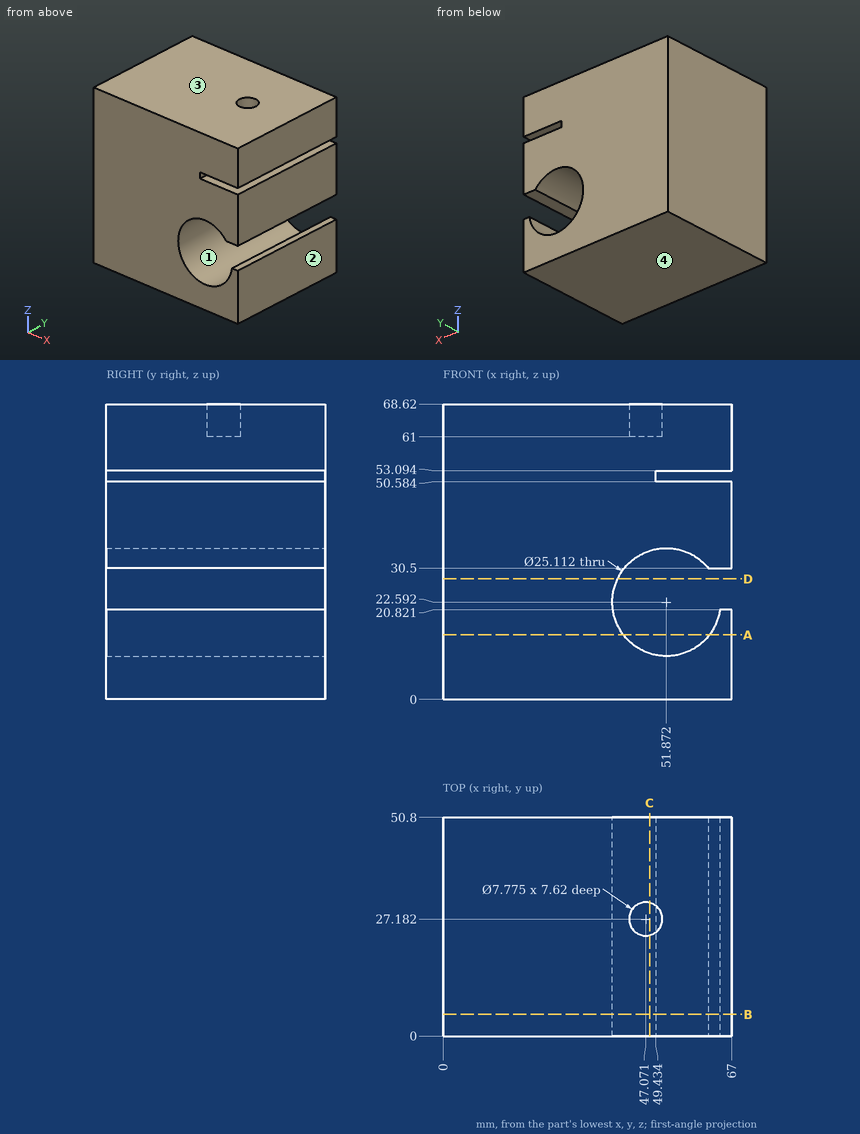
The figure shows three views and two pictorial views of one solid part (mm, origin at its lowest corner). Answer the questions. Round coordinates to 2 decimals unless told otherwise and drop trailing zeros. Order: outer loops, then holes, each group sorted by start corner. A loop starts at its lowest first (then second) coordinate and runs counter-clockwise, first axis right, second up. Notation, with made-up numbers: M 24,34 L 72,34 A27 ccw 72,67 Z; hole C -32,72.5 d3. An arc over 180 degrees is marked long. Answer in a Markdown table with one row per item. Add a question column.
1) Consider line 1 along Z through (x, y) = (51.5, 18) (1 decimal); line 2 along Z through (x, y) = (53.5, 9) (1 decimal); line 3 along X through (y, z) = (40, 32) (1 decimal). Determine where each line is inside the solid, lowest interval first. Write a range as from..to.
2) The part is cut by section C-C on x = 48. Determine the outline of the cut face in (y, z), plus the area to 4 significant figures.
3) Flat-ended cylindrical pins translate along their axes: pin 1 Ø22.5 at (x, z) = (51.87, 22.59) entering from -Y; pin 2 Ø4 at (x, y) = (46.5, 28.5) entering from +Z. Find the tip coordinate at first contact, or state that the pin passes through.
4) The part is cut by section A-A on z = 15. Determine the outline of the cut face in (x, y).
5) The part is cut by section D-D on z = 28. Determine the outline of the cut face in (x, y), plus the area to 3 significant figures.
6) The part is cut by section B-B on y = 5. Determine the outline of the cut face in (x, z) (1 decimal), plus the area to 3 significant figures.
7) Determine the mould class of the marked faces 1, 2, 3 and 4 for opening direction Z: pulls with the +Z half, pulls with the -Z half, needs draft (parallel to the pull), parting line crosses it, or undercut.
Findings below:
| question | item | result |
|---|---|---|
| 1 | line 1 | z = 0..10, 35.1..50.6, 53.1..68.6 |
| 1 | line 2 | z = 0..10.1, 35..50.6, 53.1..68.6 |
| 1 | line 3 | x = 0..43.6, 60.2..67 |
| 2 | outline | M 0,0 L 50.8,0 L 50.8,10.65 L 0,10.65 Z; M 0,34.54 L 50.8,34.54 L 50.8,68.62 L 30.96,68.62 L 30.96,61 L 23.41,61 L 23.41,68.62 L 0,68.62 Z |
| 2 | area | 2,215 mm² |
| 3 | pin 1 | passes through |
| 3 | pin 2 | stops at z = 61 |
| 4 | outline | M 0,0 L 41.87,0 L 41.87,50.8 L 0,50.8 Z; M 61.87,0 L 67,0 L 67,50.8 L 61.87,50.8 Z |
| 5 | outline | M 0,0 L 40.54,0 L 40.54,50.8 L 0,50.8 Z |
| 5 | area | 2,060 mm² |
| 6 | outline | M 0,0 L 67,0 L 67,20.8 L 64.3,20.8 A12.6 cw long 61.6,30.5 L 67,30.5 L 67,50.6 L 49.4,50.6 L 49.4,53.1 L 67,53.1 L 67,68.6 L 0,68.6 Z |
| 6 | area | 4,030 mm² |
| 7 | face 1 | undercut |
| 7 | face 2 | needs draft |
| 7 | face 3 | pulls with the +Z half |
| 7 | face 4 | pulls with the -Z half |
